The figure shows three views and two pictorial views of one solid part (mm, origin at its lowest corner). Answer the questions. A direction names the side the tool comes from. Round coordinates to 2 decimals unless told otherwise and drop trailing zeros. Order: outer loops, then holes, each group sorted by start corner. A loop starts at its lowest first (then second) coordinate and runs counter-clockwise, first axis right, second up. Notation, with made-up numbers: (72.25, 1) - (101.25, 1) arc R18 cw to (101.25, 16) - close; hole circle Ø8 at (-27.5, 78). An arc over 180 degrees is marked (long way). Answer in a Markdown table with one row per item.
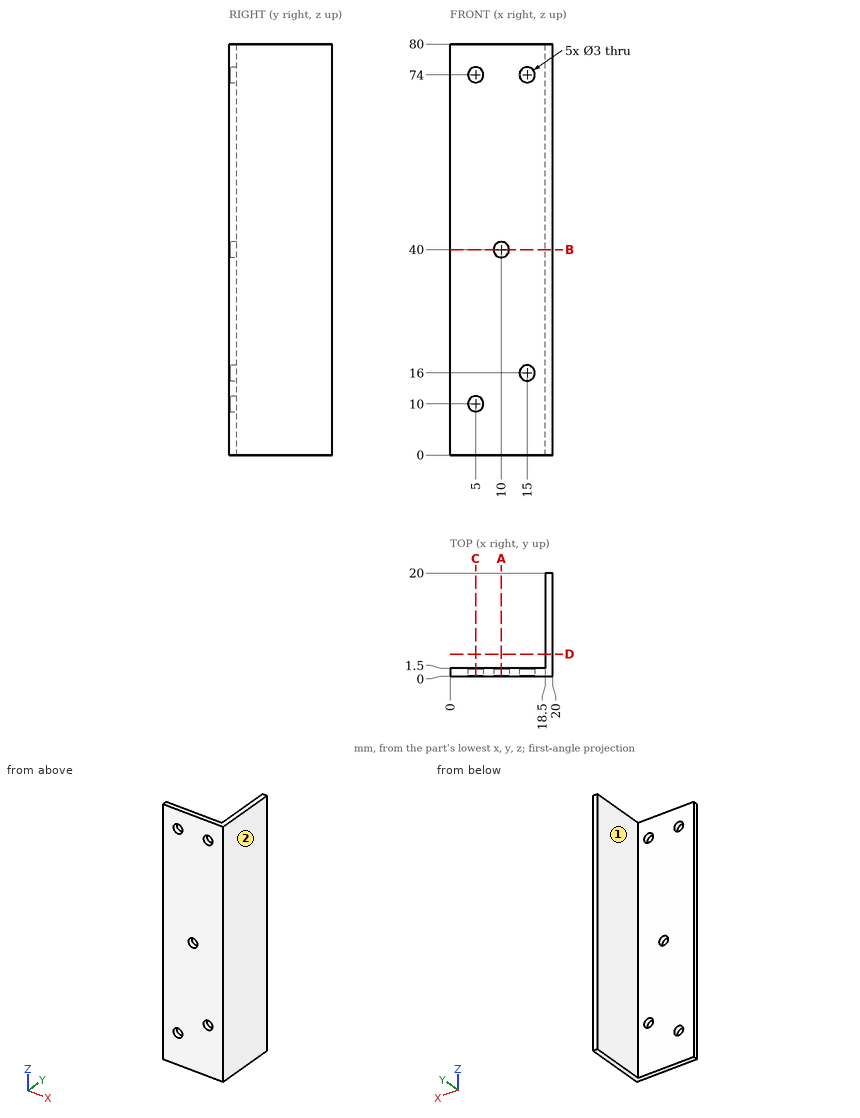
1) Find section B-B, the plane z = 40. Give the vertices of the cut face in (x, y).
Filled in:
| item | result |
|---|---|
| outline | (0, 0) - (8.5, 0) - (8.5, 1.5) - (0, 1.5) - close; (11.5, 0) - (20, 0) - (20, 20) - (18.5, 20) - (18.5, 1.5) - (11.5, 1.5) - close |
2) Find section D-D, the plane y = 4.25. Give the vertices of the cut face in (x, z).
Filled in:
| item | result |
|---|---|
| outline | (18.5, 0) - (20, 0) - (20, 80) - (18.5, 80) - close |
3) Find section A-A, the plane x = 10. Give the vertices of the cut face in (y, z).
Filled in:
| item | result |
|---|---|
| outline | (0, 0) - (1.5, 0) - (1.5, 38.5) - (0, 38.5) - close; (0, 41.5) - (1.5, 41.5) - (1.5, 80) - (0, 80) - close |
4) Each of these flat-tipped pins is pushed along its axis until it touches: pin 1 (2.5 mm diameter, centred on x = 5, z = 74, fed in from +Y); pin 2 (9 mm diameter, centred on y = 11.5, z = 34, fed in from -X); pin 3 (9 mm diameter, centred on x = 9.5, z = 46, fed in from +Y). Where does it stop, or does it pass through?
Filled in:
| item | result |
|---|---|
| pin 1 | passes through |
| pin 2 | stops at x = 18.5 |
| pin 3 | stops at y = 1.5 |
5) Find the intervals of material crossed by probe 1 along X at (y, z) = (0.95, 40); probe 2 along X at (y, z) = (1.2, 16); probe 3 along X at (y, z) = (4.5, 45), in increasing order. Write a range as from..to.
Filled in:
| item | result |
|---|---|
| probe 1 | x = 0..8.5, 11.5..20 |
| probe 2 | x = 0..13.5, 16.5..20 |
| probe 3 | x = 18.5..20 |
6) Which of the six approach directions +Z, -Z, +X, -X, +Y, -Y give full straight-line access (tool end or side, diameter ignored) to the marked faces 1 and 2?
Filled in:
| item | result |
|---|---|
| face 1 | +Z, -Z, -X, +Y |
| face 2 | +Z, -Z, +X, +Y, -Y |
7) Find section C-C, the plane x = 5. Give the vertices of the cut face in (y, z), then the cut area to 3 significant figures.
Filled in:
| item | result |
|---|---|
| outline | (0, 0) - (1.5, 0) - (1.5, 8.5) - (0, 8.5) - close; (0, 11.5) - (1.5, 11.5) - (1.5, 72.5) - (0, 72.5) - close; (0, 75.5) - (1.5, 75.5) - (1.5, 80) - (0, 80) - close |
| area | 111 mm^2 |
